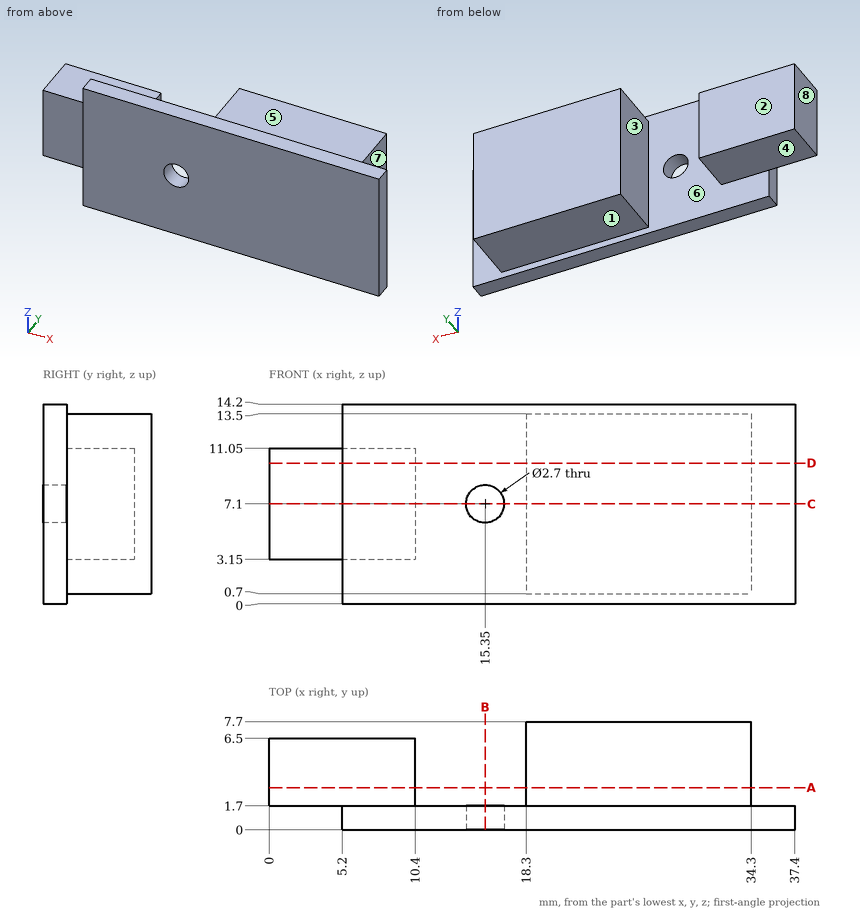
Can you work these out from the drawing? Everything is in mm from the part's minimum corner. A direction names the side the tool comes from. Give positions to 0.01 mm unless a question says otherwise; leave off trailing zeros. Loops run counter-clockwise (first coordinate to the right, second up) from the corner with the lowest first, then second, coordinate; pieces in that order, holes last. Notation, with made-up numbers: (20, 8) -> (52, 8) arc R35 cw to (52, 40) -> close; hole circle Ø10 at (26, -37.75). An arc over 180 degrees is marked (long way). Write item = value, one per line.
1) Thinking about a two-plate mould opening in X: for the marked faces 5, 6, 7 and 8, which applies, released by +X, released by -X, zero draft, split by the parting line, or undercut?
Check result:
face_5 = zero draft
face_6 = undercut
face_7 = released by +X
face_8 = released by -X
2) Suppose I cut it at D-D on z = 10. Write out the boundary of the cut face in (x, y), then the cut area to 3 significant figures.
Check result:
outline = (0, 1.7) -> (5.2, 1.7) -> (5.2, 0) -> (37.4, 0) -> (37.4, 1.7) -> (34.3, 1.7) -> (34.3, 7.7) -> (18.3, 7.7) -> (18.3, 1.7) -> (10.4, 1.7) -> (10.4, 6.5) -> (0, 6.5) -> close
area = 201 mm2
3) Suppose I cut it at C-C on z = 7.1. Write out the boundary of the cut face in (x, y), then the cut area to 3 significant figures.
Check result:
outline = (0, 1.7) -> (5.2, 1.7) -> (5.2, 0) -> (14, 0) -> (14, 1.7) -> (10.4, 1.7) -> (10.4, 6.5) -> (0, 6.5) -> close; (16.7, 0) -> (37.4, 0) -> (37.4, 1.7) -> (34.3, 1.7) -> (34.3, 7.7) -> (18.3, 7.7) -> (18.3, 1.7) -> (16.7, 1.7) -> close
area = 196 mm2
4) I need wall thicknesses on L1, parallel to X at y = 5.25, z = 10; L2, parallel to X at y = 0.75, z = 7.1; L3, parallel to Z at x = 15.5, y = 0.75. Which ranges of each line are inside material? Lowest first, please. Write a range as from..to.
Check result:
L1 = 0..10.4, 18.3..34.3
L2 = 5.2..14, 16.7..37.4
L3 = 0..5.76, 8.44..14.2
5) Will these pins go through, and if not, where does the flat tip stop? pin 1 (4 mm diameter, centred on x = 8.5, y = 4.5, fed in from -Z); pin 2 (8.5 mm diameter, centred on x = 4, z = 6.5, fed in from +Y); pin 3 (4 mm diameter, centred on y = 4, z = 7.5, fed in from +X); pin 4 (4 mm diameter, centred on x = 15.5, y = 6, fed in from -Z).
Check result:
pin_1 = 3.15
pin_2 = 6.5
pin_3 = 34.3
pin_4 = through
6) Suppose I cut it at B-B on x = 15.35. Write out the boundary of the cut face in (y, z).
Check result:
outline = (0, 0) -> (1.7, 0) -> (1.7, 5.75) -> (0, 5.75) -> close; (0, 8.45) -> (1.7, 8.45) -> (1.7, 14.2) -> (0, 14.2) -> close
7) For the marked faces 1, 2, 3 and 4, which set-ups out of +Z, -Z, +X, -X, +Y, -Y let a thin tool reach every point of the face, with its end or its side?
Check result:
face_1 = -Z, +X, -X, +Y
face_2 = +Z, -Z, -X, +Y
face_3 = +Z, -Z, +Y
face_4 = -Z, -X, +Y
8) Suppose I cut it at A-A on y = 3. Write out the boundary of the cut face in (x, z), then the cut area to 3 significant figures.
Check result:
outline = (0, 3.15) -> (10.4, 3.15) -> (10.4, 11.05) -> (0, 11.05) -> close; (18.3, 0.7) -> (34.3, 0.7) -> (34.3, 13.5) -> (18.3, 13.5) -> close
area = 287 mm2
